Verification items for the finished model (mm, model axes). Coordinates: 2 decimals unless noted, no trailing zeros. Order: outer loops, then holes, each group sorted by start corner. A loop starts at its lowest first (then second) coordinate and runs counter-clockwise, first axis right, second up. Notation, with made-up numbers: M 43.25,65 L 52.25,65 A9 cw 52.25,73 Z; hole C 22.25,37 d3. An arc over 180 degrees is marked long. Write item = value, one per line.
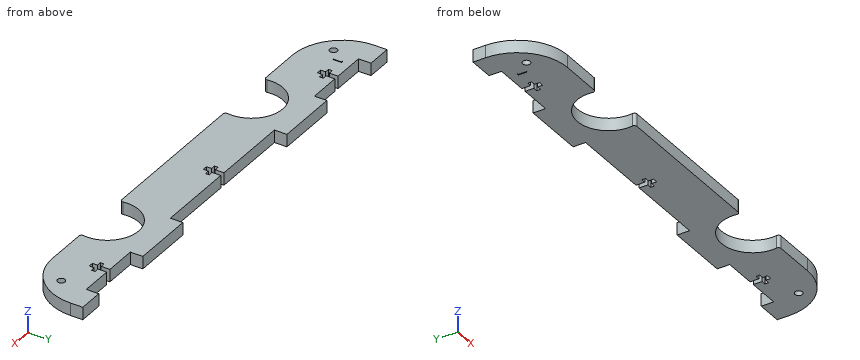
```python
from build123d import *

# Parameters (mm, degrees)
RESSALTO_EXTRUS_O1_DEPTH = 5
ESBO_O2_R                = 12.5
CORTE_EXTRUS_O1_DEPTH    = 10
FILETE2_R                = 1
ESBO_O3_W                = 27.5
ESBO_O3_H                = 5
ESBO_O3_W_2              = 65
CORTE_EXTRUS_O3_DEPTH    = 6
CORTE_EXTRUS_O4_DEPTH    = 6
ESBO_O6_R                = 1.5
CORTE_EXTRUS_O5_DEPTH    = 6


with BuildPart() as part:
    # Esboço1 → Ressalto-extrusão1 (new body)
    with BuildSketch(Plane.XY):
        with BuildLine():
            Line((20, 0), (170, 0))
            ThreePointArc((170, 0), (184.142135624, 5.857864376), (190, 20))
            Line((190, 20), (190, 25))
            Line((190, 25), (0, 25))
            Line((0, 25), (0, 20))
            ThreePointArc((0, 20), (5.857864376, 5.857864376), (20, 0))
        make_face()
    extrude(amount=RESSALTO_EXTRUS_O1_DEPTH)

    # Esboço2 → Corte-extrusão1 (cut)
    with BuildSketch(Plane.XY.offset(5)):
        with Locations((140, 2.8)):
            Circle(ESBO_O2_R)
        with Locations((50, 2.8)):
            Circle(ESBO_O2_R)
    extrude(amount=-CORTE_EXTRUS_O1_DEPTH, mode=Mode.SUBTRACT)

    # Filete2
    filete2_edges = [part.edges().sort_by_distance(p)[0] for p in [
        (127.817635697, 0, 2.5),
        (152.182364303, 0, 2.5),
        (37.817635697, 0, 2.5),
        (62.182364303, 0, 2.5),
    ]]
    fillet(filete2_edges, radius=FILETE2_R)

    # Esboço3 → Corte-extrusão3 (cut, through all)
    with BuildSketch(Plane.XY.offset(5)):
        with Locations((23.75, 22.5)):
            Rectangle(ESBO_O3_W, ESBO_O3_H)
        with Locations((95, 22.5)):
            Rectangle(ESBO_O3_W_2, ESBO_O3_H)
        with Locations((166.25, 22.5)):
            Rectangle(ESBO_O3_W, ESBO_O3_H)
    extrude(amount=-CORTE_EXTRUS_O3_DEPTH, mode=Mode.SUBTRACT)

    # Esboço5 → Corte-extrusão4 (cut, through all)
    with BuildSketch(Plane.XY.offset(5)):
        Polygon((22.75, 13), (22.75, 15), (20.95, 15), (20.95, 16.5), (22.75, 16.5), (22.75, 20), (24.75, 20), (24.75, 16.5), (26.55, 16.5), (26.55, 15), (24.75, 15), (24.75, 13), align=None)
        Polygon((94, 13), (94, 15), (92.2, 15), (92.2, 16.5), (94, 16.5), (94, 20), (96, 20), (96, 16.5), (97.8, 16.5), (97.8, 15), (96, 15), (96, 13), align=None)
        Polygon((165.2510001, 13), (165.2510001, 15), (163.4510001, 15), (163.4510001, 16.5), (165.2510001, 16.5), (165.2510001, 20), (167.2510001, 20), (167.2510001, 16.5), (169.0510001, 16.5), (169.0510001, 15), (167.2510001, 15), (167.2510001, 13), align=None)
    extrude(amount=-CORTE_EXTRUS_O4_DEPTH, mode=Mode.SUBTRACT)

    # Esboço6 → Corte-extrusão5 (cut, through all)
    with BuildSketch(Plane.XY.offset(5)):
        with Locations((180, 10)):
            Circle(ESBO_O6_R)
        with Locations((10, 10)):
            Circle(ESBO_O6_R)
        Polygon((14.350226907, 16.471731735), (14.997362324, 16.471731735), (14.997362324, 12.971731735), (14.68325976, 12.971731735), (14.68325976, 16.112757376), (14.144798222, 16.112757376), align=None)
    extrude(amount=-CORTE_EXTRUS_O5_DEPTH, mode=Mode.SUBTRACT)


solid = part.part
```
Item 1: Sectioned sample at B-B, the plane x = 140. Enter the section's corners in (y, z), then the cut area to 3 significant figures.
Report:
outline = M 15.3,0 L 25,0 L 25,5 L 15.3,5 Z
area = 48.5 mm^2
Item 2: Scan lines: L1, parallel to X at y = 7.5, z = 2.4; L2, parallel to X at y = 9.5, z = 4.5; L3, parallel to X at y = 2.8, z = 3.1. Record each from-to range of solid material in increasing order. Write a range as from..to.
Report:
L1 = 4.39..38.42, 61.58..128.42, 151.58..185.61
L2 = 2.98..8.59, 11.41..39.45, 60.55..129.45, 150.55..178.59, 181.41..187.02
L3 = 9.79..37.5, 62.5..127.5, 152.5..180.21
Item 3: Sectioned sample at D-D, the plane x = 33.5. Enter the section's corners in (y, z).
Report:
outline = M 0,0 L 20,0 L 20,5 L 0,5 Z
Item 4: Sectioned sample at A-A, the plane y = 2.8. Enter the section's corners in (x, z).
Report:
outline = M 9.79,0 L 37.5,0 L 37.5,5 L 9.79,5 Z; M 62.5,0 L 127.5,0 L 127.5,5 L 62.5,5 Z; M 152.5,0 L 180.21,0 L 180.21,5 L 152.5,5 Z
Item 5: Gauge pin test, flat ends, axial feed: pin 1 (1 mm diameter, centred on x = 165, z = 1, fed in from +Y); pin 2 (0.6 mm diameter, centred on x = 23.5, z = 3, fed in from +Y); pin 3 (0.8 mm diameter, centred on y = 16, z = 3, fed in from -X). Record the tip position at first contact, or that the pin passes through.
Report:
pin_1 = 20
pin_2 = 13
pin_3 = 0.33
Item 6: Sectioned sample at C-C, the plane z = 1.8. Give the number of separate pieces and of enclosed holes in the cut face, then the cut area to 3 significant figures.
Report:
separate_pieces = 1
enclosed_holes = 3
area = 3,270 mm^2
